```python
from build123d import *

# Parameters (mm, degrees)
SKETCH2_R           = 5.15
SKETCH2_R_2         = 11.1
BOSS_EXTRUDE2_DEPTH = 7.5


with BuildPart() as part:
    # Sketch2 → Boss-Extrude2 (new, symmetric)
    with BuildSketch(Plane(origin=(0, 0, 0), x_dir=(1, 0, 0), z_dir=(0, 1, 0))):
        with BuildLine():
            Line((-43.5, 9), (-75, 9))
            ThreePointArc((-75, 9), (-84, 0), (-75, -9))
            Line((-75, -9), (-43.5, -9))
            Line((-43.5, -9), (-2.099515649, -14.852341029))
            ThreePointArc((-2.099515649, -14.852341029), (15, 0), (-2.099515649, 14.852341029))
            Line((-2.099515649, 14.852341029), (-43.5, 9))
        make_face()
        with Locations(Location((-75, 0, 0), (0, 0, 270))):
            Circle(SKETCH2_R, mode=Mode.SUBTRACT)
        with Locations(Location((0, 0, 0), (0, 0, 270))):
            Circle(SKETCH2_R_2, mode=Mode.SUBTRACT)
    extrude(amount=BOSS_EXTRUDE2_DEPTH, both=True)


solid = part.part
```
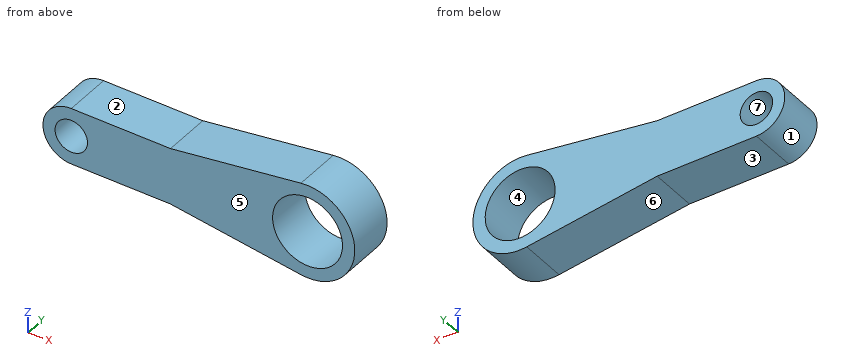
Design review of the part built by this model. Coordinates are the model's own, in mm. Face numbers are marked on the shaded views. A direction names the side the tool comes from. Coordinates: 2 decimals unless noted, no trailing zeros. Order: outer loops, then holes, each group sorted by start corner. A loop starts at its lowest first (then second) coordinate and runs counter-clockwise, first axis right, second up. Notation, with made-up numbers: (-22.75, 3) - (6.25, 3) arc R18 ccw to (6.25, 7) - close; hole circle Ø2 at (-29.75, -36.75). An arc over 180 degrees is marked (long way). Answer in a Markdown table with one row per item.
(1) Consider section D-D on z = 10. State the section outline as (x, y) points, plus the area to 3 significant figures.
Checked values:
| item | result |
|---|---|
| outline | (-36.43, -7.5) - (-4.82, -7.5) - (-4.82, 7.5) - (-36.43, 7.5) - close; (4.82, -7.5) - (11.18, -7.5) - (11.18, 7.5) - (4.82, 7.5) - close |
| area | 570 mm^2 |
(2) Clearance check with flat-ended pins moving along their axes: pin 1 (12 mm diameter, centred on x = -75, z = 0, fed in from +Y); pin 2 (2 mm diameter, centred on y = -2.5, z = 1.5, fed in from +X); pin 3 (1 mm diameter, centred on y = 2, z = -11, fed in from +X); pin 4 (1.5 mm diameter, centred on x = -63.5, y = -4.5, fed in from -Z). State where each tip first meets the part, or that it passes through.
Checked values:
| item | result |
|---|---|
| pin 1 | y = 7.5 |
| pin 2 | x = 14.99 |
| pin 3 | x = 10.71 |
| pin 4 | z = -9 |
(3) Wall thickness on line 1 along X through (y, z) = (-0.75, 0); line 2 along X through (y, z) = (-1.5, 1); line 3 along Z through (x, y) = (-46, 2.5): over which ranges is each line inside the solid? List them lowest first. Write a range as from..to.
Checked values:
| item | result |
|---|---|
| line 1 | -84..-80.15, -69.85..-11.1, 11.1..15 |
| line 2 | -83.94..-80.05, -69.95..-11.05, 11.05..14.97 |
| line 3 | -9..9 |
(4) Consider section A-A on x = 0. State the section outline as (y, z) points, plus the area to 3 significant figures.
Checked values:
| item | result |
|---|---|
| outline | (-7.5, -15) - (7.5, -15) - (7.5, -11.1) - (-7.5, -11.1) - close; (-7.5, 11.1) - (7.5, 11.1) - (7.5, 15) - (-7.5, 15) - close |
| area | 117 mm^2 |
(5) Consider section B-B on z = 0. State the section outline as (x, y) points.
Checked values:
| item | result |
|---|---|
| outline | (-84, -7.5) - (-80.15, -7.5) - (-80.15, 7.5) - (-84, 7.5) - close; (-69.85, -7.5) - (-11.1, -7.5) - (-11.1, 7.5) - (-69.85, 7.5) - close; (11.1, -7.5) - (15, -7.5) - (15, 7.5) - (11.1, 7.5) - close |
(6) For the marked faces 1, 2 and 3, list the 3-axis set-ups (+Z, -Z, +X, -X, +Y, -Y) from which the entire face can be reached by the end or side of a thin tool; tool diameter is ignored.
Checked values:
| item | result |
|---|---|
| face 1 | -X, +Y, -Y |
| face 2 | +Z, -X, +Y, -Y |
| face 3 | -Z, -X, +Y, -Y |
(7) The part is to be moulded in two halves that separate along Z. For the marked faces 4, 5, 6 and 7, say which applies: released by +Z, released by -Z, zero draft, split by the parting line, or undercut.
Checked values:
| item | result |
|---|---|
| face 4 | undercut |
| face 5 | zero draft |
| face 6 | released by -Z |
| face 7 | undercut |
(8) Consider section C-C on y = -3.25. State the section outline as (x, z) points.
Checked values:
| item | result |
|---|---|
| outline | (-75, -9) - (-43.5, -9) - (-2.1, -14.85) arc R15 ccw (long way) to (-2.1, 14.85) - (-43.5, 9) - (-75, 9) arc R9 ccw to start; hole circle Ø10.3 at (-75, 0); hole circle Ø22.2 at (0, 0) |
